from build123d import *

# Parameters (mm, degrees)
F0_W      = 160
F0_H      = 150
F1_DEPTH  = 86
F3_DEPTH  = 20
F4_W      = 20
F4_H      = 14
F5_DEPTH  = 2
F6_R      = 2.5
F7_DEPTH  = 2
F8_R      = 1
F9_DEPTH  = 25
F10_W     = 23
F10_H     = 32
F11_DEPTH = 10
F12_R     = 65
F13_DEPTH = 5


with BuildPart() as f1:
    # F0 (on Top) → F1 (new body)
    with BuildSketch(Plane.XY):
        with Locations((93.771139, 75)):
            Rectangle(F0_W, F0_H)
    extrude(amount=F1_DEPTH)

    # F2 (on face) → F3 (cut)
    with BuildSketch(Plane.YZ.offset(173.771139)):
        Polygon((37, 53), (23, 53), (18, 48), (18, 38), (42, 38), (42, 48), align=None)
    extrude(amount=-F3_DEPTH, mode=Mode.SUBTRACT)

    # F4 (on face) → F5 (join)
    with BuildSketch(Plane.YZ.offset(173.771139)):
        with Locations((30, 66)):
            Rectangle(F4_W, F4_H)
    extrude(amount=F5_DEPTH)

    # F6 (on face) → F7 (join)
    with BuildSketch(Plane.YZ.offset(173.771139)):
        with BuildLine():
            Line((23, 56), (10.518483, 49.999966))
            ThreePointArc((10.518483, 49.999966), (5.500009, 45.009242), (10.5, 40))
            Line((10.5, 40), (23, 34))
            Line((23, 34), (37, 34))
            Line((37, 34), (49.5, 40))
            ThreePointArc((49.5, 40), (54.5, 45), (49.5, 50))
            Line((49.5, 50), (37, 56))
            Line((37, 56), (23, 56))
        make_face()
        with Locations((10.5, 45)):
            Circle(F6_R, mode=Mode.SUBTRACT)
        Polygon((42, 38), (18, 38), (18, 48), (23, 53), (37, 53), (42, 48), align=None, mode=Mode.SUBTRACT)
        with Locations((49.5, 45)):
            Circle(F6_R, mode=Mode.SUBTRACT)
    extrude(amount=F7_DEPTH)

    # F8 (on face) → F9 (cut)
    with BuildSketch(Plane.YZ.offset(173.771139)):
        with Locations((30, 80)):
            Circle(F8_R)
        with Locations((6, 6)):
            Circle(F8_R)
        with Locations((144, 70.5)):
            Circle(F8_R)
        with Locations((144, 6)):
            Circle(F8_R)
    extrude(amount=-F9_DEPTH, mode=Mode.SUBTRACT)

    # F10 (on face) → F11 (cut)
    with BuildSketch(Plane(origin=(13.771139, 0, 0), x_dir=(0, -1, 0), z_dir=(-1, 0, 0))):
        with Locations((-12.5, 49)):
            Rectangle(F10_W, F10_H)
    extrude(amount=-F11_DEPTH, mode=Mode.SUBTRACT)

    # F12 (on face) → F13 (cut)
    with BuildSketch(Plane(origin=(0, 0, 0), x_dir=(1, 0, 0), z_dir=(0, 0, -1))):
        with Locations((93.771139, -75)):
            Circle(F12_R)
    extrude(amount=-F13_DEPTH, mode=Mode.SUBTRACT)


solid = f1.part
CAD build for the part. Positions are in the model's coordinates, mm. A direction names the side the tool comes from. Coordinates: 2 decimals unless noted, no trailing zeros. Loops run counter-clockwise (first coordinate to the right, second up) from the corner with the lowest first, then second, coordinate; pieces in that order, holes last. Notation, with made-up numbers: (22.25, 81) -> (55.25, 81) arc R26 cw to (55.25, 98) -> close; hole circle Ø3 at (27.5, 15). An arc over 180 degrees is marked (long way). One line per item, written item: value.
1. Slice it at C-C on x = 139. Write the cut outline in (y, z).
Answers:
outline: (0, 0) -> (28.32, 0) -> (28.32, 5) -> (121.68, 5) -> (121.68, 0) -> (150, 0) -> (150, 86) -> (0, 86) -> close
2. Drill centre lines: line 1 (Z direction, x = 167, y = 144); line 2 (X direction, y = 99.5, z = 38); line 3 (Z direction, x = 81, y = 125). Where is each one in solid material? Low to high. Write a range as [from, to].
Answers:
line 1: z = [0, 5], [7, 69.5], [71.5, 86]
line 2: x = [13.77, 173.77]
line 3: z = [5, 86]
3. Which spindle directions (+Z, -Z, +X, -X, +Y, -Y) get a long thin tool onto all of the face, cutting with end or side? Do faces 1 (the face through (174.757, 43.162, 36.958)), 2 (the face through (174.757, 16.662, 37.042)), 3 (the face through (165, 30, 38)), 4 (the face through (155.77, 55.48, 2.46)). Say none if no direction does.
Answers:
face 1: -Z, +X, +Y
face 2: -Z, +X, -Y
face 3: +X
face 4: -Z
4. Pull direction Z, two halves, no side cores. Call faces 5 (the face through (174.8, 54.5, 44.9)), 6 (the face through (93, 76, 86)), 7 (the face through (19, 13, 65)), 8 (the face through (13.771, 74, 42)): pulls with the +Z half, pulls with the -Z half, needs draft (parallel to the pull), parting line crosses it, or undercut.
Answers:
face 5: parting line crosses it
face 6: pulls with the +Z half
face 7: undercut
face 8: needs draft
5. Slice it at A-A on z = 45. Write the cut outline in (x, y).
Answers:
outline: (13.77, 0) -> (173.77, 0) -> (173.77, 5.5) -> (175.77, 5.5) -> (175.77, 8) -> (173.77, 8) -> (173.77, 13) -> (175.77, 13) -> (175.77, 18) -> (153.77, 18) -> (153.77, 42) -> (175.77, 42) -> (175.77, 47) -> (173.77, 47) -> (173.77, 52) -> (175.77, 52) -> (175.77, 54.5) -> (173.77, 54.5) -> (173.77, 150) -> (13.77, 150) -> (13.77, 24) -> (23.77, 24) -> (23.77, 1) -> (13.77, 1) -> close
6. Slice it at B-B on y = 137. Write the cut outline in (x, z), and give its area (3 significant figures).
Answers:
outline: (13.77, 0) -> (74.25, 0) -> (74.25, 5) -> (113.29, 5) -> (113.29, 0) -> (173.77, 0) -> (173.77, 86) -> (13.77, 86) -> close
area: 13,600 mm^2
7. Flat gauge pins, fed straight in: P1, Ø12, axis at x = 36, z = 45, coming from the -Y side; P2, Ø1, axis at y = 28, z = 13.5, coming from the +X side; P3, Ø5, axis at x = 136.5, y = 119.5, coming from the -Z side; P4, Ø8, axis at y = 10.5, z = 45, coming from the -X side. Where does each tip first touch, or does it go through?
Answers:
P1: stops at y = 0
P2: stops at x = 173.77
P3: stops at z = 5
P4: stops at x = 23.77
